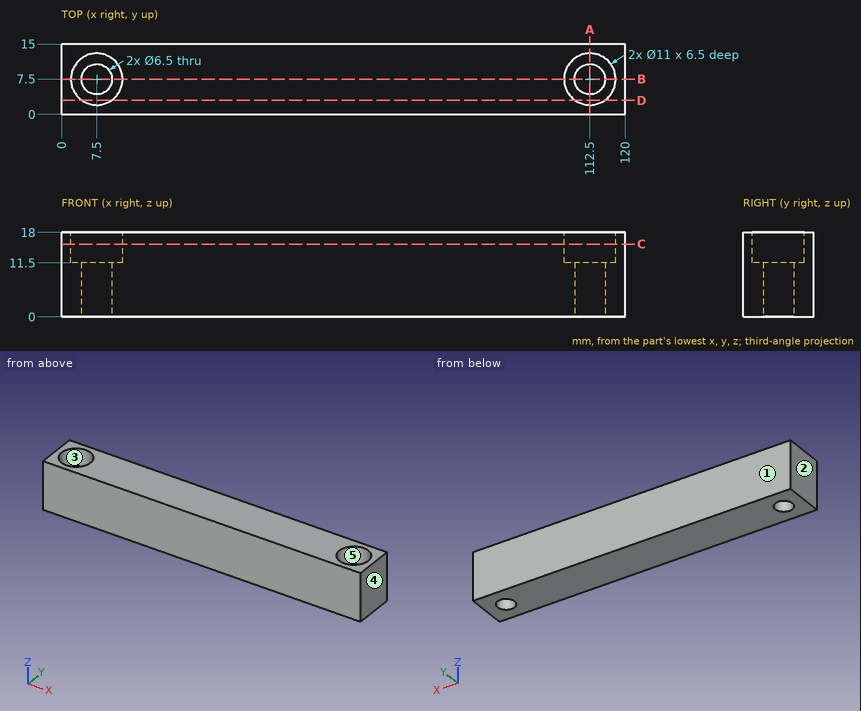
Can you work these out from the drawing? Everything is in mm from the part's minimum corner. A direction names the side the tool comes from. Give positions to 0.01 mm unless a question says otherwise; leave off trailing zeros. Loops run counter-clockwise (first coordinate to the right, second up) from the corner with the lowest first, then second, coordinate; pieces in that order, holes last. Notation, with made-up numbers: (-34, 24.5) -> (-20, 24.5) arc R25 cw to (-20, 56.5) -> close; hole circle Ø4 at (-8, -14.5). An arc over 180 degrees is marked (long way). Return JSON: item names as keys, results as strings.
Item 1: I'm going to push a flat-ended pin straight in: pin 1 (5.5 mm diameter, centred on x = 111, y = 9, fed in from +Z). Where does the tip first touch, or does it pass through?
Geometry results:
{"pin 1": "stops at z = 11.5"}
Item 2: If we section it at A-A on x = 112.5: List the corners of the cut face in (y, z) for me.
Geometry results:
{"outline": "(0, 0) -> (4.25, 0) -> (4.25, 11.5) -> (2, 11.5) -> (2, 18) -> (0, 18) -> close; (10.75, 0) -> (15, 0) -> (15, 18) -> (13, 18) -> (13, 11.5) -> (10.75, 11.5) -> close"}
Item 3: If we section it at D-D on y = 3: List the corners of the cut face in (x, z) for me, plus the area to 3 significant figures.
Geometry results:
{"outline": "(0, 0) -> (120, 0) -> (120, 18) -> (115.66, 18) -> (115.66, 11.5) -> (109.34, 11.5) -> (109.34, 18) -> (10.66, 18) -> (10.66, 11.5) -> (4.34, 11.5) -> (4.34, 18) -> (0, 18) -> close", "area": "2,080 mm²"}
Item 4: I need wall thicknesses on L1, parallel to X at y = 7.75, z = 9.25; L2, parallel to X at y = 7, z = 12.75; L3, parallel to Z at x = 115.5, y = 3. Which ranges of each line are inside material? Lowest first, please. Write a range as from..to.
Geometry results:
{"L1": "x = 0..4.26, 10.74..109.26, 115.74..120", "L2": "x = 0..2.02, 12.98..107.02, 117.98..120", "L3": "z = 0..11.5"}
Item 5: Which directions (+Z, -Z, +X, -X, +Y, -Y) give clear straight access to the entire face, cutting with the end or side of a thin tool? Please do the marked faces 4 and 5.
Geometry results:
{"face 4": "+Z, -Z, +X, +Y, -Y", "face 5": "+Z"}
Item 6: If we section it at C-C on z = 15.5: List the corners of the cut face in (x, y) for me, plus the area to 3 significant figures.
Geometry results:
{"outline": "(0, 0) -> (120, 0) -> (120, 15) -> (0, 15) -> close; hole circle Ø11 at (7.5, 7.5); hole circle Ø11 at (112.5, 7.5)", "area": "1,610 mm²"}
Item 7: If we section it at B-B on y = 7.5: List the corners of the cut face in (x, z) for me.
Geometry results:
{"outline": "(0, 0) -> (4.25, 0) -> (4.25, 11.5) -> (2, 11.5) -> (2, 18) -> (0, 18) -> close; (10.75, 0) -> (109.25, 0) -> (109.25, 11.5) -> (107, 11.5) -> (107, 18) -> (13, 18) -> (13, 11.5) -> (10.75, 11.5) -> close; (115.75, 0) -> (120, 0) -> (120, 18) -> (118, 18) -> (118, 11.5) -> (115.75, 11.5) -> close"}
Item 8: We'd pull the mould along Y, two halves only. Please class the marked faces 1, 2 and 3: +Y half, -Y half, draft (parallel to the pull), parting line (faces both ways), or undercut.
Geometry results:
{"face 1": "+Y half", "face 2": "draft", "face 3": "undercut"}
